```python
from build123d import *

# Parameters (mm, degrees)
ESQUISSE1_R        = 1.55
ESQUISSE1_R_2      = 4
ESQUISSE1_R_3      = 1.35255
ESQUISSE1_R_4      = 2.7051
BOSS_EXTRU_1_DEPTH = 3


with BuildPart() as part:
    # Esquisse1 → Boss.-Extru.1 (new body)
    with BuildSketch(Plane(origin=(0, 0, 0), x_dir=(0, 0, -1), z_dir=(1, 0, 0))):
        with BuildLine():
            Line((-40.60825, -12.7), (-40.60825, -16.144875))
            Line((-40.60825, -16.144875), (-40.60825, -16.348305132))
            add(Edge.make_bspline(
                [(-40.60825, -16.348305132), (-40.365634485, -16.661193605), (-40.112338127, -16.96547542), (-39.63020507, -17.593748723), (-39.400688032, -17.917191992), (-38.719045939, -18.893089111), (-38.271947044, -19.549593057), (-37.338540998, -20.831006808), (-36.855460104, -21.458516341), (-36.059725811, -22.342477591), (-35.781944124, -22.627029047), (-35.202868212, -23.17718548), (-34.900674383, -23.443503751), (-33.971943166, -24.212706181), (-33.324405882, -24.685383849), (-32.010805282, -25.604549776), (-31.348089528, -26.055770333), (-30.303090708, -26.660610546), (-29.948270215, -26.848696892), (-29.222483721, -27.184971005), (-28.851412004, -27.333773538), (-28.083597976, -27.570691368), (-27.685315555, -27.657976057), (-27.090666934, -27.715403346), (-26.891908645, -27.722631025), (-26.592836888, -27.712936491), (-26.492990431, -27.706278992), (-26.292963936, -27.685632014), (-26.192732932, -27.670522326), (-26.092449031, -27.65425)],
                knots=[0, 0, 0, 0, 0.0625, 0.0625, 0.125, 0.125, 0.25, 0.25, 0.375, 0.375, 0.4375, 0.4375, 0.5, 0.5, 0.625, 0.625, 0.75, 0.75, 0.8125, 0.8125, 0.875, 0.875, 0.9375, 0.9375, 0.96875, 0.96875, 0.984375, 0.984375, 1, 1, 1, 1], degree=3))
            Line((-26.092449031, -27.65425), (-26.092449031, -90))
            ThreePointArc((-26.092449031, -90), (2.64551669, -116.14013034), (25.954024412, -85.06135051))
            Line((25.954024412, -85.06135051), (25.954024412, -27.65425))
            add(Edge.make_bspline(
                [(25.954024412, -27.65425), (27.179118802, -27.419536533), (28.353377808, -27.051803075), (30.05705383, -26.34918771), (30.615126485, -26.089288473), (31.712904721, -25.521429223), (32.254485024, -25.212118815), (33.827204106, -24.230350536), (34.814025463, -23.502087852), (36.672007358, -21.907218093), (37.543320305, -21.040793316), (38.751902771, -19.623473398), (39.134714509, -19.134962989), (39.851014333, -18.131439591), (40.185535135, -17.615291382), (40.801362362, -16.550595558), (41.082635497, -16.002027673), (41.457015911, -15.150237789), (41.574249194, -14.86042264), (41.789713906, -14.277065554), (41.888049248, -13.98351322), (42.334688534, -12.506770959), (42.546239761, -11.296312151), (42.717568356, -9.451511475), (42.750611649, -8.83067761), (42.772859866, -7.900507946), (42.775360474, -7.590422151), (42.77555993, -6.970221998), (42.772087252, -6.66010067), (42.772087252, -6.35)],
                knots=[0, 0, 0, 0, 0.125, 0.125, 0.1875, 0.1875, 0.25, 0.25, 0.375, 0.375, 0.5, 0.5, 0.5625, 0.5625, 0.625, 0.625, 0.6875, 0.6875, 0.71875, 0.71875, 0.75, 0.75, 0.875, 0.875, 0.9375, 0.9375, 0.96875, 0.96875, 1, 1, 1, 1], degree=3))
            add(Edge.make_bspline(
                [(42.772087252, -6.35), (42.772087252, -5.874878454), (42.783792207, -5.398095979), (42.789657917, -4.447020546), (42.781867467, -3.973004463), (42.672546396, -2.563152451), (42.499179213, -1.637510108), (42.106282017, -0.267897459), (41.954068536, 0.185625042), (41.614819435, 1.087728793), (41.430081297, 1.530283034), (40.844911495, 2.839259084), (40.416604561, 3.689518781), (39.046783283, 6.190525131), (38.013123304, 7.787251584), (36.291657446, 10.082106977), (35.688509547, 10.830664164), (34.43654182, 12.281738953), (33.786199883, 12.985690235), (33.112075, 13.668565083)],
                knots=[0, 0, 0, 0, 0.0625, 0.0625, 0.125, 0.125, 0.25, 0.25, 0.3125, 0.3125, 0.375, 0.375, 0.5, 0.5, 0.75, 0.75, 0.875, 0.875, 1, 1, 1, 1], degree=3))
            add(Edge.make_bspline(
                [(33.112075, 13.668565083), (32.332207955, 14.539101946), (31.435060987, 15.277734234)],
                knots=[0, 0, 0, 1, 1, 1], degree=2))
            add(Edge.make_bspline(
                [(31.435060987, 15.277734234), (30.299691041, 16.309376592), (29.113704516, 17.275445235), (26.646604831, 19.084346085), (25.360475951, 19.928267183), (21.432297769, 22.265681686), (18.70167828, 23.563722979), (14.477833082, 25.213127628), (13.049229105, 25.71486416), (10.864398428, 26.369911185), (10.129061703, 26.571832136), (8.64156399, 26.936524394), (7.890831572, 27.098844789), (5.637990782, 27.512412208), (4.127431428, 27.693727696), (2.225306731, 27.768676851), (1.844136038, 27.775542931), (1.080940786, 27.779973661), (0.698904769, 27.777413484), (-0.446346689, 27.779064109), (-1.208874123, 27.797823926), (-2.732682239, 27.815308111), (-3.492085471, 27.806304753), (-5.004084105, 27.739990771), (-5.756994671, 27.684916502), (-8.006157922, 27.451797552), (-9.492662784, 27.204583891), (-11.701987236, 26.688775277), (-12.434852331, 26.491461598), (-13.894254142, 26.051929085), (-14.622118919, 25.807493497), (-16.765417144, 25.01223388), (-18.151500369, 24.400517874), (-20.847821735, 23.032525232), (-22.158708475, 22.277484827), (-24.716496252, 20.645447351), (-25.966430559, 19.7652326), (-28.39125747, 17.919703458), (-29.567431908, 16.954258357), (-31.287557173, 15.454109034), (-31.85380584, 14.945666112), (-32.972832423, 13.91291508), (-33.52577931, 13.388805977), (-34.066096443, 12.849822171)],
                knots=[0, 0, 0, 0, 0.0625, 0.0625, 0.125, 0.125, 0.25, 0.25, 0.3125, 0.3125, 0.34375, 0.34375, 0.375, 0.375, 0.4375, 0.4375, 0.453125, 0.453125, 0.46875, 0.46875, 0.5, 0.5, 0.53125, 0.53125, 0.5625, 0.5625, 0.625, 0.625, 0.65625, 0.65625, 0.6875, 0.6875, 0.75, 0.75, 0.8125, 0.8125, 0.875, 0.875, 0.9375, 0.9375, 0.96875, 0.96875, 1, 1, 1, 1], degree=3))
            add(Edge.make_bspline(
                [(-34.066096443, 12.849822171), (-35.159801618, 11.692162737), (-36.251081621, 10.53740284), (-37.166580532, 9.404947171)],
                knots=[0, 0, 0, 0, 1, 1, 1, 1], degree=3))
            ThreePointArc((-37.166580532, 9.404947171), (-37.363014685, 9.160281042), (-37.557796616, 8.914297524))
            add(Edge.make_bspline(
                [(-37.557796616, 8.914297524), (-38.142933539, 8.170182683), (-38.709522845, 7.412667282), (-39.741912272, 5.824816801), (-40.203133529, 4.998794666), (-40.60825, 4.142494902)],
                knots=[0, 0, 0, 0, 0.5, 0.5, 1, 1, 1, 1], degree=3))
            Line((-40.60825, 4.142494902), (-40.60825, -12.7))
        make_face()
        with Locations((0.1651, -103.128774516)):
            Circle(ESQUISSE1_R, mode=Mode.SUBTRACT)
        with Locations((-12.963674516, -90)):
            Circle(ESQUISSE1_R, mode=Mode.SUBTRACT)
        with Locations((0.1651, -90)):
            Circle(ESQUISSE1_R_2, mode=Mode.SUBTRACT)
        with Locations((0.1651, -76.871225484)):
            Circle(ESQUISSE1_R, mode=Mode.SUBTRACT)
        with Locations((13.293874516, -90)):
            Circle(ESQUISSE1_R, mode=Mode.SUBTRACT)
        with Locations((-16.9799, -14.9225)):
            Circle(ESQUISSE1_R_3, mode=Mode.SUBTRACT)
        with Locations((0.1651, -18.2245)):
            Circle(ESQUISSE1_R_4, mode=Mode.SUBTRACT)
        with Locations((0.1651, 6.103472306)):
            Circle(ESQUISSE1_R_3, mode=Mode.SUBTRACT)
        with Locations((17.3101, -14.9225)):
            Circle(ESQUISSE1_R_3, mode=Mode.SUBTRACT)
    extrude(amount=BOSS_EXTRU_1_DEPTH)


solid = part.part
```
Can you work these out from the model? Positions are in its coordinate system, mm. A direction names the side the tool comes from. Round coordinates to 2 decimals unless told otherwise and drop trailing zeros. Loops run counter-clockwise (first coordinate to the right, second up) from the corner with the lowest first, then second, coordinate; pieces in that order, holes last.
Item 1: Suppose I cut it at A-A, the plane y = -72.5. Write out the boundary of the cut face in (x, z), then the cut area to 3 significant figures.
Item 2: Which directions (+Z, -Z, +X, -X, +Y, -Y) give clear straight access to the entire face, cutting with the end or side of a thin tool? Please do faces 4 (the flat face through (1, -57, -25.954)), 5 (the cylindrical face through (1.479, -20.865, 0.421)).
Item 3: Please list where these lines run through material, in increasing order: L1, parallel to Z at x = 2.05, y = -89; L2, parallel to Z at x = 0.15, y = -69.5; L3, parallel to Z at x = 2, y = -16.5.
Item 4: Will these pins go through, and if not, where does the flat tip stop? pin 1 Ø0.9 at (x, y) = (1, -45) entering from -Z; pin 2 Ø2.5 at (y, z) = (6.1, -0.17) entering from -X; pin 3 Ø1.5 at (x, z) = (2.5, 10.5) entering from -Y.
Item 5: If we mould it in two halves opening along Z, with no side actions, what happens to faces 1 (the cylindrical face through (1.48, -13.58, -17.13)), 2 (the cylindrical face through (1.48, -116.19, -2.04)), 3 (the flat face through (1, -6, 40.608))? For each: +Z half, -Z half, draft (parallel to the pull), parting line (faces both ways), or undercut.
Item 6: Suppose I cut it at B-B, the plane x = 1.8. State how many separate pieces and enclosed holes the cut face has, then the cut area to 3 significant figures.
Reported:
1. outline: (0, -25.95) - (3, -25.95) - (3, 26.09) - (0, 26.09) - close
1. area: 156 mm2
2. face 4: -Z, +X, -X
2. face 5: +X, -X
3. L1: z = -26.4 to -14.48, -12.11 to -4.04, 3.71 to 11.78, 14.15 to 26.09
3. L2: z = -25.95 to 26.09
3. L3: z = -40.82 to -2.25, 1.92 to 40.49
4. pin 1: stops at z = -25.95
4. pin 2: passes through
4. pin 3: stops at y = -114.31
5. face 1: undercut
5. face 2: parting line
5. face 3: +Z half
6. separate pieces: 1
6. enclosed holes: 9
6. area: 8,070 mm2
